```python
from build123d import *

# Parameters (mm, degrees)
SKETCH1_R           = 75
BOSS_EXTRUDE1_DEPTH = 645
SKETCH2_W           = 150
SKETCH2_H           = 645
BOSS_EXTRUDE2_DEPTH = 1290
FILLET1_R           = 65


with BuildPart() as part:
    # Sketch1 → Boss-Extrude1 (new body)
    with BuildSketch(Plane.XY):
        with Locations(Location((0, 0, 0), (0, 0, 180))):
            Circle(SKETCH1_R)
    extrude(amount=BOSS_EXTRUDE1_DEPTH)

    # Sketch2 → Boss-Extrude2 (add)
    with BuildSketch(Plane(origin=(0, 0, 0), x_dir=(1, 0, 0), z_dir=(0, 1, 0))):
        with Locations((0, -322.5)):
            Rectangle(SKETCH2_W, SKETCH2_H)
    extrude(amount=BOSS_EXTRUDE2_DEPTH)

    # Fillet1
    fillet1_edges = [part.edges().sort_by_distance(p)[0] for p in [
        (-75, 645, 645),
        (75, 645, 645),
        (-75, 1290, 322.5),
        (0, 1290, 645),
        (75, 1290, 322.5),
        (0, 1290, 0),
        (0, -75, 645),
    ]]
    fillet(fillet1_edges, radius=FILLET1_R)


solid = part.part
```
Verification items for the finished model (mm, model axes). Round coordinates to 2 decimals unless told otherwise and drop trailing zeros. Write each loop counter-clockwise with the first axis right and the second up, starting at its lowest first coordinate (ties: lowest second). Pieces come first, ordered by that corner, then holes. Notation, with made-up numbers: (34, 62.25) -> (86, 62.25) arc R13 cw to (86, 68.25) -> close; hole circle Ø1 at (40, 8.25). An arc over 180 degrees is marked (long way). Write each question's results on one line, items separated by ' | '. Start each with the question number.
1. Depth check by flat-ended pin: P1, Ø4, axis at x = 16.5, z = 544, coming from the +Y side; P2, Ø3, axis at x = -17.5, z = 84, coming from the -Y side; P3, Ø5, axis at x = -43.5, z = 455, coming from the +Y side. Enter the tip coordinate at first touch or a pass-through.
2. Material ranges on probe 1 along Z at (x, y) = (-16, 229); probe 2 along X at (y, z) = (-5.5, 393.5); probe 3 along Z at (x, y) = (-15, -1), recorded low to high. Write a range as from..to.
3. Cross-section at A-A (y = 154.5). Enter the section's corners in (x, z).
4. Cross-section at B-B (z = 279). Enter the section's corners in (x, y), then the cut area to 3 significant figures.
Solutions:
1) P1: stops at y = 1289.84 | P2: stops at y = -73.27 | P3: stops at y = 1282.13
2) probe 1: z = 0..644.72 | probe 2: x = -74.8..74.8 | probe 3: z = 0..644.8
3) outline: (-75, 0) -> (75, 0) -> (75, 580) arc R65 ccw to (10, 645) -> (-10, 645) arc R65 ccw to (-75, 580) -> close
4) outline: (-75, 0) arc R75 ccw to (75, 0) -> (75, 1225) arc R65 ccw to (10, 1290) -> (-10, 1290) arc R65 ccw to (-75, 1225) -> close | area: 201,000 mm2
